Can you work these out from the model? Positions are in its coordinate system, mm. A direction names the side the tool comes from. Give positions to 0.01 mm unless a question says otherwise; leave off trailing zeros. Loops run counter-clockwise (first coordinate to the right, second up) from the corner with the lowest first, then second, coordinate; pieces in that order, holes last. Notation, with made-up numbers: (23.25, -36.5) - (76.25, -36.5) arc R29 cw to (76.25, -12.5) - close; hole circle Ø1 at (-2, -14.5). An arc over 180 degrees is marked (long way). Answer as a JSON object with one key per item and string values. Group by question number.
Item 1: Which directions (+Z, -Z, +X, -X, +Y, -Y) give clear straight access to the entire face, cutting with the end or side of a thin tool? Please do faces 5 (the flat face through (0, 0, -80)), 6 (the flat face through (0, 10, -59)), 7 (the flat face through (-10, 0, -59)).
Item 2: Will these pins go through, and if not, where does the flat tip stop? pin 1 (10 mm diameter, centred on y = 4.5, z = -94, fed in from -X); pin 2 (12 mm diameter, centred on x = 8, z = -62.5, fed in from -Y); pin 3 (11 mm diameter, centred on x = -40, y = -33, fed in from -Z); pin 4 (18 mm diameter, centred on x = 40, y = -33, fed in from -Z).
Item 3: Suppose I cut it at B-B on y = 33. Write out the boundary of the cut face in (x, z), and give its area (3 significant figures).
Item 4: Thinking about a two-plate mould opening in X: for faces 1 (the flat face through (0, -10, -59)), 2 (the flat face through (5, 0, -93)), 3 (the flat face through (-5, 0, -93)), 4 (the flat face through (-60, -1, 5)), which applies, pulls with the +X half, pulls with the -X half, needs draft (parallel to the pull), parting line crosses it, or undercut?
Item 5: Suppose I cut it at D-D on y = -43.5. Write out the boundary of the cut face in (x, z), and give its area (3 significant figures).
Item 6: Please list where these lines run through material, in increasing order: L1, parallel to Y at x = -40, z = 7.5; L2, parallel to X at y = -4, z = -102.5; L3, parallel to Z at x = 3, y = 2.
Item 7: Suppose I cut it at C-C on x = -1. Write out the boundary of the cut face in (y, z), and give its area (3 significant figures).
Item 8: Suppose I cut it at A-A on x = -40. Write out the boundary of the cut face in (y, z).
from build123d import *

# Parameters (mm, degrees)
F0_W     = 20
F0_H     = 20
F2_DEPTH = 120
F0_W_2   = 120
F0_H_2   = 106
F0_R     = 7
F3_DEPTH = 10
F1_W     = 10
F1_H     = 25
F4_DEPTH = 12.5


with BuildPart() as f2:
    # F0 (on Top) → F2 (new body)
    with BuildSketch(Plane.XY):
        Rectangle(F0_W, F0_H)
    extrude(amount=-F2_DEPTH)

    # F0 (on Top) → F3 (join)
    with BuildSketch(Plane.XY):
        Rectangle(F0_W_2, F0_H_2)
        with Locations((-40, -33)):
            Circle(F0_R, mode=Mode.SUBTRACT)
        with Locations((40, -33)):
            Circle(F0_R, mode=Mode.SUBTRACT)
        with Locations((-40, 33)):
            Circle(F0_R, mode=Mode.SUBTRACT)
        Rectangle(F0_W, F0_H, mode=Mode.SUBTRACT)
        with Locations((40, 33)):
            Circle(F0_R, mode=Mode.SUBTRACT)
        Rectangle(F0_W, F0_H)
    extrude(amount=F3_DEPTH)

    # F1 (on Front) → F4 (cut, symmetric)
    with BuildSketch(Plane.XZ):
        with Locations((0, -92.5)):
            Rectangle(F1_W, F1_H)
    extrude(amount=F4_DEPTH, both=True, mode=Mode.SUBTRACT)


solid = f2.part
Worked out:
{
 "1": {"face 5": "+Y, -Y", "face 6": "-Z, +X, -X, +Y", "face 7": "-Z, -X, +Y, -Y"},
 "2": {"pin 1": "stops at x = -10", "pin 2": "stops at y = -10", "pin 3": "passes through", "pin 4": "stops at z = 0"},
 "3": {"outline": "(-60, 0) - (-47, 0) - (-47, 10) - (-60, 10) - close; (-33, 0) - (33, 0) - (33, 10) - (-33, 10) - close; (47, 0) - (60, 0) - (60, 10) - (47, 10) - close", "area": "920 mm2"},
 "4": {"face 1": "needs draft", "face 2": "undercut", "face 3": "undercut", "face 4": "pulls with the -X half"},
 "5": {"outline": "(-60, 0) - (60, 0) - (60, 10) - (-60, 10) - close", "area": "1,200 mm2"},
 "6": {"L1": "y = -53 to -40, -26 to 26, 40 to 53", "L2": "x = -10 to -5, 5 to 10", "L3": "z = -120 to -105, -80 to 10"},
 "7": {"outline": "(-53, 0) - (-10, 0) - (-10, -80) - (10, -80) - (10, 0) - (53, 0) - (53, 10) - (-53, 10) - close; (-10, -120) - (10, -120) - (10, -105) - (-10, -105) - close", "area": "2,960 mm2"},
 "8": {"outline": "(-53, 0) - (-40, 0) - (-40, 10) - (-53, 10) - close; (-26, 0) - (26, 0) - (26, 10) - (-26, 10) - close; (40, 0) - (53, 0) - (53, 10) - (40, 10) - close"}
}
